Autodesk Inventor part; units mm, degrees
ref_plane "YZ Plane" through (0, 0, 0) normal (1, 0, 0) x (0, 1, 0)
ref_plane "XZ Plane" through (0, 0, 0) normal (0, 1, 0) x (-1, 0, 0)
ref_plane "XY Plane" through (0, 0, 0) normal (0, 0, 1) x (1, 0, 0)
sketch "Sketch1" plane through (0, 0, 0) normal (0, 0, 1) x (1, 0, 0)
  line L0 (-46.7038, 15.5679) -> (443.2962, 15.5679)
  line L1 (443.2962, 15.5679) -> (443.2962, -95.4321)
  line L2 (443.2962, -95.4321) -> (-46.7038, -95.4321)
  line L3 (-46.7038, -95.4321) -> (-46.7038, 15.5679)
  point P0 (0, 0)
  dimension "d0" = 490
  dimension "d1" = 111
extrude "Extrusion1" add sketch "Sketch1" along normal blind 15
sketch "Sketch2" plane through (443.2962, -95.4321, 0) normal (1, 0, 0) x (0, 0, -1)
  line L0 (0, 0) -> (0, 111)
  line L1 (0, 111) -> (-5, 111)
  line L2 (-5, 111) -> (-5, 0)
  line L3 (-5, 0) -> (0, 0)
  line L4 (0, 0) -> (0, 111)
  point P0 (0, 95.4321)
  dimension "d4" = 5
  dimension "d5" = 111
extrude "Extrusion2" cut sketch "Sketch2" against normal blind 7
sketch "Sketch3" plane through (-46.7038, -95.4321, 0) normal (-1, 0, 0) x (0, 0, 1)
  line L0 (0, 111) -> (0, 0)
  line L1 (0, 111) -> (5, 111)
  line L2 (5, 111) -> (5, 0)
  line L3 (5, 0) -> (0, 0)
  line L4 (0, 0) -> (0, 111)
  point P0 (0, 95.4321)
  dimension "d8" = 5
  dimension "d9" = 111
extrude "Extrusion3" cut sketch "Sketch3" against normal blind 7
sketch "Sketch4" plane through (0, 0, 0) normal (0, 0, -1) x (-1, 0, 0)
  line L0 (-436.2962, 15.5679) -> (-436.2962, -95.4321)
  line L1 (-436.2962, 15.5679) -> (39.7038, 15.5679)
  line L2 (39.7038, 15.5679) -> (39.7038, 5.5679)
  line L3 (39.7038, 5.5679) -> (-436.2962, 5.5679)
  line L4 (-436.2962, 5.5679) -> (-436.2962, 15.5679)
  point P0 (0, 0)
  dimension "d12" = 476
  dimension "d13" = 10
extrude "Extrusion4" cut sketch "Sketch4" against normal blind 5
sketch "Sketch5" plane through (0, 0, 0) normal (0, 0, -1) x (-1, 0, 0)
  line L0 (39.7038, 5.5679) -> (-436.2962, 5.5679)
  line L1 (-436.2962, 5.5679) -> (-436.2962, -95.4321)
  line L2 (39.7038, -95.4321) -> (-436.2962, -95.4321)
  line L3 (39.7038, -95.4321) -> (39.7038, 5.5679)
  line L4 (-436.2962, -95.4321) -> (-436.2962, 5.5679)
  line L5 (39.7038, 5.5679) -> (39.7038, -95.4321)
  line L6 (-436.2962, 5.5679) -> (39.7038, 5.5679)
  line L7 (39.7038, 5.5679) -> (39.7038, -95.4321)
  line L8 (39.7038, -95.4321) -> (-436.2962, -95.4321)
  line L9 (-436.2962, -95.4321) -> (-436.2962, 5.5679)
  point P0 (0, 0)
extrude "Extrusion5" add sketch "Sketch5" along normal blind 1
properties part number "Arcade_FrontBottom"
The model under review builds one solid part; all positions refer to its coordinate system, in mm. Round coordinates to 2 decimals unless told otherwise and drop trailing zeros. Loops run counter-clockwise (first coordinate to the right, second up) from the corner with the lowest first, then second, coordinate; pieces in that order, holes last. Notation, with made-up numbers: (25, -18) -> (39, -18) arc R28 ccw to (39, 16) -> close; hole circle Ø6 at (45, 66). An arc over 180 degrees is marked (long way). Return JSON: item names as keys, results as strings.
(1) Add section A-A on x = 55. Write out the cut boundary in (y, z).
Solved:
{"outline": "(-95.43, -1) -> (5.57, -1) -> (5.57, 5) -> (15.57, 5) -> (15.57, 15) -> (-95.43, 15) -> close"}
(2) For line 1 (Z direction, x = 417, y = 6.5); line 2 (Y direction, x = 404.5, z = 1); line 3 (X direction, y = -33, z = 3.5), list the stretches that pass through material, from the lowest coordinate up.
Solved:
{"line 1": "5 to 15", "line 2": "-95.43 to 5.57", "line 3": "-39.7 to 436.3"}
(3) For pin 1 (5 mm diameter, centred on y = -43.5, z = 2, fed in from +X); pin 2 (5 mm diameter, centred on y = -40.5, z = 0.5, fed in from -X), all flat-tipped, find the tip position at first contact; note any pin that passes through.
Solved:
{"pin 1": "x = 436.3", "pin 2": "x = -39.7"}
